Verification items for the finished model (mm, model axes). Face numbers are marked on the shaded views. Coordinates: 2 decimals unless noted, no trailing zeros. Order: outer loops, then holes, each group sorted by start corner. A loop starts at its lowest first (then second) coordinate and runs counter-clockwise, first axis right, second up.
Q1. Depth check by flat-ended pin: P1, Ø8.5, axis at x = 0, z = 0, coming from the -Y side. Enter the tip coordinate at first touch or a pass-through.
Q2. Cross-section at A-A, the plane x = 0. Record the boundary of the cut face in (y, z) (1 decimal), and give its area (3 significant figures).
Q3. Draft check along X on the marked faces 1, 2 and 3. Enter one of: pulls with the +X half, pulls with the -X half, needs draft (parallel to the pull), parting line crosses it, or undercut.
Q4. Cross-section at B-B, the plane z = 0. Record the boundary of the cut face in (x, y) (1 decimal).
Q5. Thickness scan on line 1 (Z direction, x = 0, y = 1.8) (3 decimals); line 2 (X direction, y = 1.85, z = 0) (3 decimals); line 3 (X direction, y = 2.45, z = -3) (3 decimals). Record the ranges inside material, lowest first.
Q6. Cross-section at D-D, the plane z = 16.5. Record the boundary of the cut face in (x, y).
from build123d import *

# Parameters (mm, degrees)
SKETCH1_W           = 69.85
SKETCH1_H           = 44.45
BOSS_EXTRUDE1_DEPTH = 4.7625
SKETCH2_R           = 7.14375
CUT_EXTRUDE1_DEPTH  = 5.7625
FILLET1_R           = 19.05
FILLET2_R           = 19.05


with BuildPart() as part:
    # Sketch1 → Boss-Extrude1 (new body)
    with BuildSketch(Plane(origin=(0, 0, 0), x_dir=(1, 0, 0), z_dir=(0, 1, 0))):
        Rectangle(SKETCH1_W, SKETCH1_H)
    extrude(amount=BOSS_EXTRUDE1_DEPTH)

    # Sketch2 → Cut-Extrude1 (cut, through all)
    with BuildSketch(Plane(origin=(0, 4.7625, 0), x_dir=(1, 0, 0), z_dir=(0, 1, 0))):
        Circle(SKETCH2_R)
    extrude(amount=-CUT_EXTRUDE1_DEPTH, mode=Mode.SUBTRACT)

    # Fillet1
    fillet1_edges = [part.edges().sort_by_distance(p)[0] for p in [
        (-34.925, 2.38125, 22.225),
        (-34.925, 2.38125, -22.225),
    ]]
    fillet(fillet1_edges, radius=FILLET1_R)

    # Fillet2
    fillet2_edges = [part.edges().sort_by_distance(p)[0] for p in [
        (34.925, 2.38125, 22.225),
        (34.925, 2.38125, -22.225),
    ]]
    fillet(fillet2_edges, radius=FILLET2_R)


solid = part.part
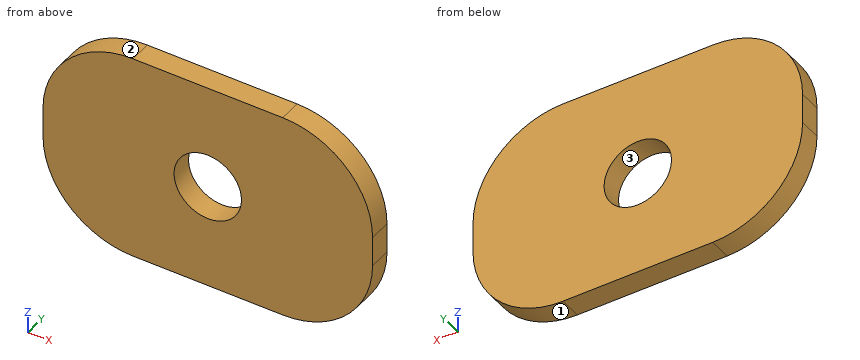
Check values:
1. P1: passes through
2. outline: (0, -22.2) - (4.8, -22.2) - (4.8, -7.1) - (0, -7.1) - close; (0, 7.1) - (4.8, 7.1) - (4.8, 22.2) - (0, 22.2) - close
2. area: 144 mm2
3. face 1: pulls with the +X half
3. face 2: pulls with the -X half
3. face 3: undercut
4. outline: (-34.9, 0) - (-7.1, 0) - (-7.1, 4.8) - (-34.9, 4.8) - close; (7.1, 0) - (34.9, 0) - (34.9, 4.8) - (7.1, 4.8) - close
5. line 1: z = -22.225 to -7.144, 7.144 to 22.225
5. line 2: x = -34.925 to -7.144, 7.144 to 34.925
5. line 3: x = -34.925 to -6.483, 6.483 to 34.925
6. outline: (-29.49, 0) - (29.49, 0) - (29.49, 4.76) - (-29.49, 4.76) - close
